For this review, take the finished solid that the model builds, in its own axes (mm). A direction names the side the tool comes from. Give positions to 0.01 mm unless a question says otherwise; leave off trailing zeros. Write each loop counter-clockwise with the first axis right and the second up, starting at its lowest first coordinate (ties: lowest second). Pieces come first, ordered by that corner, then holes.
from build123d import *

# Parameters (mm, degrees)
SKETCH_1_R      = 2.25
SKETCH_1_R_2    = 32.5
EXTRUDE_1_DEPTH = 32.9


with BuildPart() as part:
    # 草图1 → 凸台-拉伸1 (new body)
    with BuildSketch(Plane(origin=(0, 0, 0), x_dir=(1, 0, 0), z_dir=(0, 1, 0))):
        with BuildLine():
            Line((32.038228151, 34.251451604), (36.985161154, 37.464270068))
            ThreePointArc((36.985161154, 37.464270068), (42.395709987, 36.811885931), (42.716072869, 31.371572396))
            Line((42.716072869, 31.371572396), (38.645559751, 26.573120094))
            ThreePointArc((38.645559751, 26.573120094), (32.742735514, -33.578613299), (-27.538659341, -37.96356466))
            ThreePointArc((-27.538659341, -37.96356466), (-34.46083935, -40.331140059), (-33.202224105, -33.12434625))
            ThreePointArc((-33.202224105, -33.12434625), (-40.995709816, -22.780732575), (-45.663114217, -10.7))
            Line((-45.663114217, -10.7), (-49.7, -10.7))
            Line((-49.7, -10.7), (-49.7, 46.9))
            Line((-49.7, 46.9), (0, 46.9))
            ThreePointArc((0, 46.9), (17.222324463, 43.623405875), (32.038228151, 34.251451604))
        make_face()
        with Locations(Location((-31.7, -37.1, 0), (0, 0, 270))):
            Circle(SKETCH_1_R, mode=Mode.SUBTRACT)
        with Locations(Location((39.3, 33.9, 0), (0, 0, 270))):
            Circle(SKETCH_1_R, mode=Mode.SUBTRACT)
        with Locations(Location((0, -4.7, 0), (0, 0, 270))):
            Circle(SKETCH_1_R_2, mode=Mode.SUBTRACT)
    extrude(amount=EXTRUDE_1_DEPTH)


solid = part.part
(1) We need section D-D (x = 35.5). Write out the cut boundary in (y, z), and give its area (3 significant figures).
(2) Tool access review of faces 4 (the flat face through (40.709, 16.22, -29.006)), 5 (the flat face through (-48, 16, 10.7)), 6 (the cylindrical face through (16.992, 16.22, -43.713)): name each direction out of +Z, -Z, +X, -X, +Y, -Y from which nothing blocks a thin tool from reaching the whole face with its end or side.
(3) We need section C-C (y = 30.5). Write out the cut boundary in (x, z).
(4) We need section B-B (z = -3). Write out the cut boundary in (x, y), and give its area (3 significant figures).
(5) We need section A-A (x = 23). Write out the cut boundary in (y, z).
(6) For L1, parallel to X at y = 23.5, z = -35; L2, parallel to X at y = 22.5, z = -33.9; L3, parallel to X at y = 20.5, z = -30, list the stretches that pass through material, from the lowest coordinate up.
(7) The part is to be moulded in two halves that separate along X. For faces 1 (the flat face through (-25, 16, -46.9)), 2 (the cylindrical face through (37.931, 16.22, -35.686)), 3 (the flat face through (-49.7, 16, -18)), say which applies: +X half, -X half, draft (parallel to the pull), parting line (faces both ways), or undercut.
(8) Clearance check with flat-ended pins moving along their axes: pin 1 Ø2.5 at (x, z) = (39.3, -33.9) entering from +Y; pin 2 Ø4 at (y, z) = (14, -23.5) entering from +X; pin 3 Ø1.2 at (x, y) = (-47, 16.5) entering from +Z; pin 4 Ø8 at (x, y) = (-1.5, 14) entering from +Z. State where each tip first meets the part, or that it passes through.
The answers:
1. outline: (0, -36.5) - (32.9, -36.5) - (32.9, 30.65) - (0, 30.65) - close
1. area: 2,210 mm2
2. face 4: +X, +Y, -Y
2. face 5: +Z, -X, +Y, -Y
2. face 6: -Z, +Y, -Y
3. outline: (-49.7, -46.9) - (0, -46.9) arc R46.9 ccw to (32.04, -34.25) - (36.99, -37.46) arc R4.25 ccw to (42.72, -31.37) - (38.65, -26.57) arc R46.9 ccw to (-27.54, 37.96) arc R4.25 ccw (long way) to (-33.2, 33.12) arc R46.9 ccw to (-45.66, 10.7) - (-49.7, 10.7) - close; hole circle Ø4.5 at (-31.7, 37.1); hole circle Ø65 at (0, 4.7); hole circle Ø4.5 at (39.3, -33.9)
4. outline: (-49.7, 0) - (-31.57, 0) - (-31.57, 32.9) - (-49.7, 32.9) - close; (31.57, 0) - (46.8, 0) - (46.8, 32.9) - (31.57, 32.9) - close
4. area: 1,100 mm2
5. outline: (0, -40.87) - (32.9, -40.87) - (32.9, -18.26) - (0, -18.26) - close; (0, 27.66) - (32.9, 27.66) - (32.9, 40.87) - (0, 40.87) - close
6. L1: x = -49.7 to 31.22, 33.19 to 37.34, 41.26 to 43.41
6. L2: x = -49.7 to 37.05, 41.55 to 43.55
6. L3: x = -49.7 to 41.55
7. face 1: draft
7. face 2: undercut
7. face 3: -X half
8. pin 1: passes through
8. pin 2: stops at x = 41.68
8. pin 3: stops at z = 10.7
8. pin 4: stops at z = 46.9
